Geometry: final body of the model. Coordinates: model frame, mm. Face numbers are marked on the shaded views. A direction names the side the tool comes from. Give positions to 0.01 mm unless a question says otherwise; leave off trailing zeros. Put each result on its own line as item: value.
```python
from build123d import *

# Parameters (mm, degrees)
F2_R     = 5.08
F3_W     = 75.227168
F3_H     = 48.306637
F4_DEPTH = 34.29


with BuildPart() as f1:
    # F0 (on Front) → F1 (revolve)
    with BuildSketch(Plane.XZ):
        with BuildLine():
            Line((-26.501408, 0), (-31.777891, 0))
            ThreePointArc((-31.777891, 0), (-24.236438, -20.553089), (-5.191517, -31.350958))
            Line((-5.191517, -31.350958), (-5.191517, -28.482988))
            Line((-5.191517, -28.482988), (-5.612337, -28.482988))
            Line((-5.612337, -28.482988), (-5.612337, -24.601767))
            Line((-5.612337, -24.601767), (-9.852801, -24.601767))
            ThreePointArc((-9.852801, -24.601767), (-21.948095, -14.852803), (-26.501408, 0))
        make_face()
    revolve(axis=Axis((0, 0, -28.432627), (0, 0, 1)))

    # F2
    f2_edges = [f1.edges().sort_by_distance(p)[0] for p in [
        (26.501408, 0, 0),
    ]]
    fillet(f2_edges, radius=F2_R)

    # F3 (on Right) → F4 (cut)
    with BuildSketch(Plane.YZ):
        with Locations((-0.6491, -24.153318)):
            Rectangle(F3_W, F3_H)
    extrude(amount=-F4_DEPTH, mode=Mode.SUBTRACT)


solid = f1.part
```
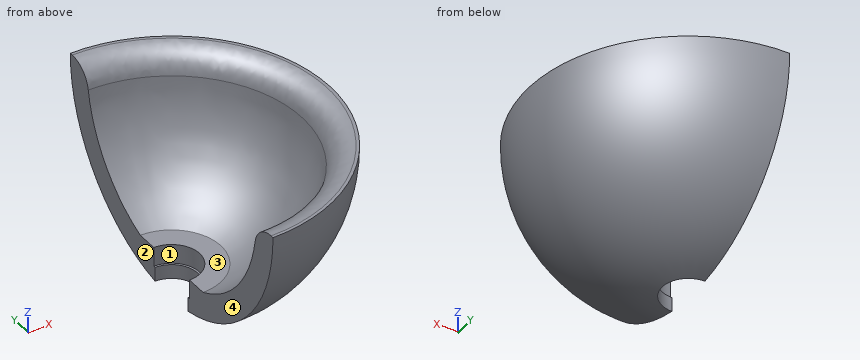
Item 1: Pin query (flat end, axial travel): pin 1 Ø6 at (x, y) = (17.5, -15.5) entering from -Z; pin 2 Ø10 at (x, z) = (27, -8.5) entering from +Y; pin 3 Ø1 at (x, y) = (21, -5) entering from -Z. Return the tip coordinate at first contact, or that it passes through.
Output values:
pin 1: z = -24.38
pin 2: y = 21.6
pin 3: z = -23.77
Item 2: Mould query, pull axis Y, two halves, no side actions, for the marked faces 3 and 4. Classes: pulls with the +Y half, pulls with the -Y half, needs draft (parallel to the pull), parting line crosses it, or undercut.
Output values:
face 3: undercut
face 4: needs draft
Item 3: Set-up query: the marked faces 1 and 2. Return all of +Z, -Z, +X, -X, +Y, -Y with unobstructed straight access to the full face (end or side cutting, diameter ignored); none if empty.
Output values:
face 1: +Z, -X
face 2: +Z, -Z, -X, +Y, -Y
Item 4: Line query: probe 1 along Y at (x, z) = (18.5, -2); probe 2 along Z at (x, y) = (11, 14); probe 3 along Z at (x, y) = (3, -28). Output: solid intervals per line, ascending. Write a range as [from, to].
Output values:
probe 1: [-25.76, -19.84], [19.84, 25.76]
probe 2: [-26.32, -19.63]
probe 3: [-14.73, -0.99]
